Geometry: final body of the model. Coordinates: model frame, mm. A direction names the side the tool comes from. Coordinates: 2 decimals unless noted, no trailing zeros. Write each loop counter-clockwise with the first axis right and the second up, starting at its lowest first coordinate (ties: lowest second). Pieces come first, ordered by that corner, then holes. Notation, with made-up numbers: (-12, -31) -> (15, -31) arc R11 ccw to (15, -17) -> close; hole circle Ø9 at (35, 70.25). An arc over 180 degrees is marked (long way). One line per item, written item: value.
```python
from build123d import *

# Parameters (mm, degrees)
PAD_DEPTH = 20


with BuildPart() as part:
    # Sketch → Pad (new body)
    with BuildSketch(Plane.YZ):
        with BuildLine():
            Line((-23, -1), (0, -1))
            ThreePointArc((0, -1), (1, 0), (0, 1))
            Line((-23, 1), (0, 1))
            ThreePointArc((-23, 1), (-24, 0), (-23, -1))
        make_face()
        with BuildLine():
            Line((-23, -0.5), (0, -0.5))
            ThreePointArc((0, -0.5), (0.5, 0), (0, 0.5))
            Line((-23, 0.5), (0, 0.5))
            ThreePointArc((-23, 0.5), (-23.5, 0), (-23, -0.5))
        make_face(mode=Mode.SUBTRACT)
    extrude(amount=PAD_DEPTH)


solid = part.part
```
(1) Pull-direction query (Z, two-part tool) for faces 3 (the flat face through (10, -12, -0.5)), 4 (the flat face through (10, -12, -1)), 5 (the flat face through (0, -11.7, 0.7)); classes: released by +Z, released by -Z, zero draft, split by the parting line, or undercut.
Responses:
face 3: undercut
face 4: released by -Z
face 5: zero draft
(2) Section C-C (x = 17.5). Return the cut outline in (y, z).
Responses:
outline: (-23, -1) -> (0, -1) arc R1 ccw to (0, 1) -> (-23, 1) arc R1 ccw to start; hole (-23, -0.5) -> (0, -0.5) arc R0.5 ccw to (0, 0.5) -> (-23, 0.5) arc R0.5 ccw to start
(3) Line query: line 1 (Z direction, x = 17, y = -17.5); line 2 (Y direction, x = 7, z = 0.4); line 3 (Y direction, x = 10.25, z = -0.05). Output: solid intervals per line, ascending. Write a range as [from, to].
Responses:
line 1: z = [-1, -0.5], [0.5, 1]
line 2: y = [-23.92, -23.3], [0.3, 0.92]
line 3: y = [-24, -23.5], [0.5, 1]
(4) Section B-B (y = -9.25). Return the cut outline in (x, z).
Responses:
outline: (0, -1) -> (20, -1) -> (20, -0.5) -> (0, -0.5) -> close; (0, 0.5) -> (20, 0.5) -> (20, 1) -> (0, 1) -> close
(5) Reachability of faces 1 (the cylindrical face through (10, -24, 0)), 2 (the cylindrical face through (9.9, -23.5, 0)) from +Z, -Z, +X, -X, +Y, -Y: full face, straight path, thin tool, end or side. Return the list, or none.
Responses:
face 1: +X, -X, -Y
face 2: +X, -X
(6) Section A-A (z = 0). Return the cut outline in (x, y).
Responses:
outline: (0, -24) -> (20, -24) -> (20, -23.5) -> (0, -23.5) -> close; (0, 0.5) -> (20, 0.5) -> (20, 1) -> (0, 1) -> close
